Check sheet for the drawn part. Datum: minimum x, y, z corner. Units: mm. A direction names the side the tool comes from. Give positions to 0.01 mm unless a question says otherwise; leave off trailing zeros. Write each loop counter-clockwise with the first axis right and the second up, starting at its lowest first coordinate (ties: lowest second). Pieces come first, ordered by that corner, then holes. Notation, with made-up numbers: (16.25, -15.75) - (60.25, -15.75) arc R18 cw to (60.25, 14.25) - close; hole circle Ø10 at (87, 55). An arc over 180 degrees is marked (long way). Return JSON: item names as keys, results as strings. Group by question number.
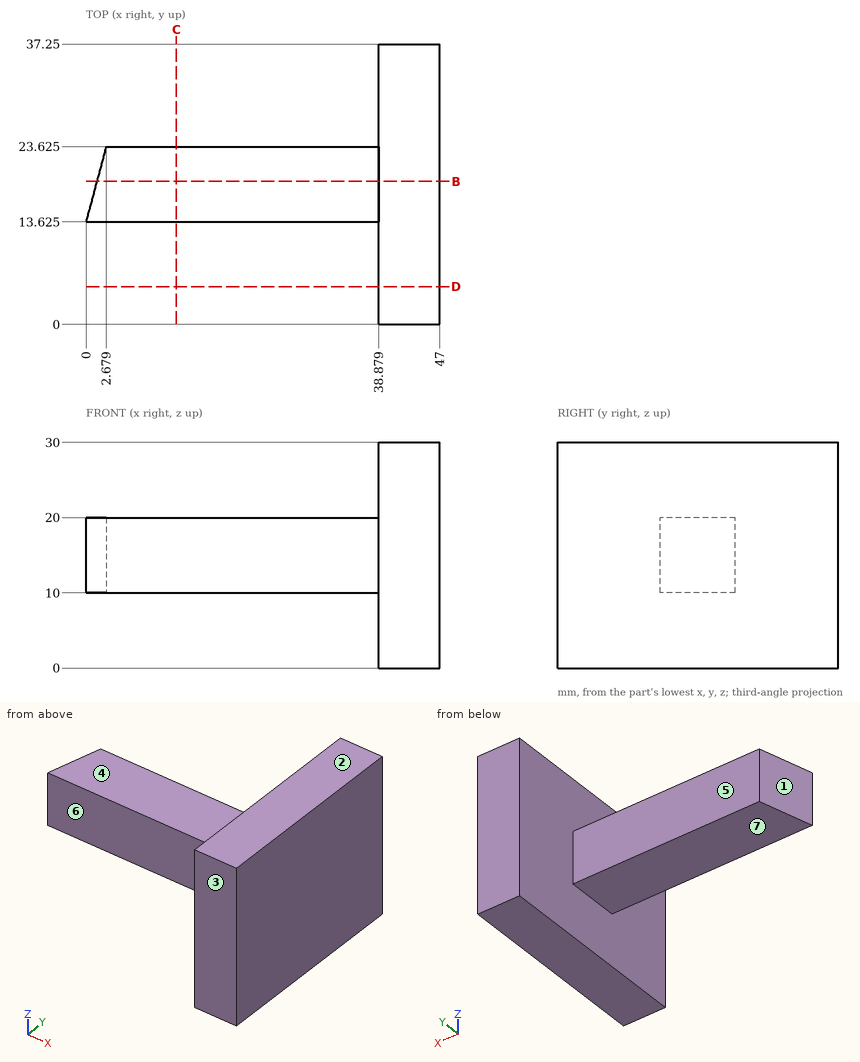
Item 1: Section check D-D on y = 5. Record the cut outline in (x, z), plus the area to 3 significant figures.
Item 2: Material ranges on line 1 along Y through (x, z) = (36.5, 19) (1 decimal); line 2 along X through (y, z) = (6.5, 1.5); line 3 along Z through (x, y) = (26.5, 17.5), recorded low to high. Write a range as from..to.
Item 3: Mould release check, pull along Y, two halves, no side actions. Record for the marked faces 1, 2 and 3: +Y half, -Y half, draft (parallel to the pull), parting line (faces both ways), or undercut.
Item 4: Depth check by flat-ended pin: pin 1 (8 mm diameter, centred on x = 14.5, z = 16, fed in from -Y) (1 decimal); pin 2 (10 mm diameter, centred on x = 13, y = 32.5, fed in from -Z); pin 3 (8 mm diameter, centred on x = 25, y = 16.5, fed in from -Z); pin 4 (3 mm diameter, centred on x = 19, z = 17.5, fed in from +Y) (1 decimal). Enter the tip coordinate at first touch or a pass-through.
Item 5: Section check B-B on y = 19. Record the cut outline in (x, z), plus the area to 3 significant figures.
Item 6: Access from +Z, -Z, +X, -X, +Y, -Y to the whole of each face (thin tool, end or side, straight path). Record for the marked faces 4, 5, 6 and 7.
Item 7: Section check C-C on x = 12. Record the cut outline in (y, z) (1 decimal).
Reply:
{
 "1": {"outline": "(38.88, 0) - (47, 0) - (47, 30) - (38.88, 30) - close", "area": "244 mm²"},
 "2": {"line 1": "13.6..23.6", "line 2": "38.88..47", "line 3": "10..20"},
 "3": {"face 1": "+Y half", "face 2": "draft", "face 3": "-Y half"},
 "4": {"pin 1": "y = 13.6", "pin 2": "through", "pin 3": "z = 10", "pin 4": "y = 23.6"},
 "5": {"outline": "(1.44, 10) - (38.88, 10) - (38.88, 0) - (47, 0) - (47, 30) - (38.88, 30) - (38.88, 20) - (1.44, 20) - close", "area": "618 mm²"},
 "6": {"face 4": "+Z, -X, +Y, -Y", "face 5": "+Z, -Z, -X, +Y", "face 6": "+Z, -Z, -X, -Y", "face 7": "-Z, -X, +Y, -Y"},
 "7": {"outline": "(13.6, 10) - (23.6, 10) - (23.6, 20) - (13.6, 20) - close"}
}
